Autodesk Inventor part; units mm, degrees
ref_plane "YZ Plane" through (0, 0, 0) normal (1, 0, 0) x (0, 1, 0)
ref_plane "XZ Plane" through (0, 0, 0) normal (0, 1, 0) x (-1, 0, 0)
ref_plane "XY Plane" through (0, 0, 0) normal (0, 0, 1) x (1, 0, 0)
sketch "スケッチ1" plane through (0, 0, 0) normal (0, 1, 0) x (-1, 0, 0)
  circle A0 centre (0, 0) radius 4
  dimension "d0" = 8
extrude "押し出し1" add sketch "スケッチ1" along normal blind 5
fillet "フィレット1" radius 0.2 1 edges at (4, 5, 0)
fillet "フィレット2" radius 0.2 1 edges at (4, 0, 0)
sketch "スケッチ2" plane through (0, 5, 0) normal (0, 1, 0) x (1, 0, 0)
  circle A0 centre (0, 0) radius 2
  dimension "d5" = 4
extrude "押し出し2" cut sketch "スケッチ2" against normal blind 5
sketch "スケッチ3" plane through (0, 0, 0) normal (0, 0, 1) x (1, 0, 0)
  line L0 (3.8, 0) -> (-3.8, 0)
  point P0 (0, 0)
  point P1 (0, 2.5)
  dimension "d8" = 2.5
hole "穴1" at (0, 2.5, 0) direction (0, 0, -1) diameter 2.459 depth 5 tip angle 118
properties part number "シャフトカラー" material "ステンレス鋼"
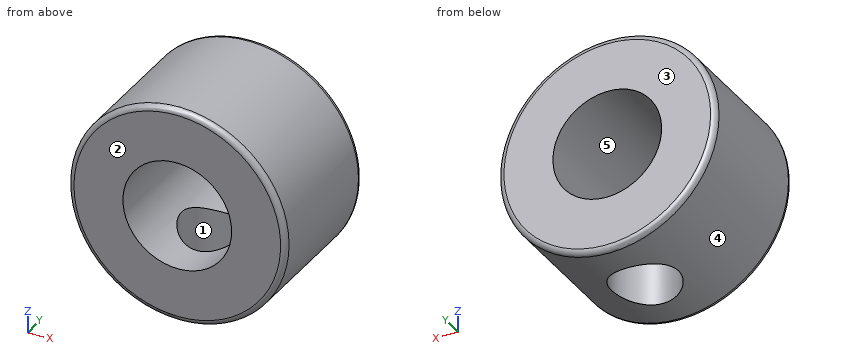
CAD build for the part. Positions are in the model's coordinates, mm. Face numbers are marked on the shaded views. A direction names the side the tool comes from. Round coordinates to 2 decimals unless told otherwise and drop trailing zeros. Order: outer loops, then holes, each group sorted by start corner. A loop starts at its lowest first (then second) coordinate and runs counter-clockwise, first axis right, second up. Notation, with made-up numbers: (34, 57.25) -> (69, 57.25) arc R8 cw to (69, 67.25) -> close; hole circle Ø8 at (38, 4.25). An arc over 180 degrees is marked (long way). One line per question, with ' | ' between items.
Q1. Two-plate mould, pull along X, no slides. Class the marked faces 3, 4 and 5: released by +X, released by -X, zero draft, split by the parting line, or undercut.
Completed:
face 3: zero draft | face 4: split by the parting line | face 5: undercut
Q2. Drop flat-ended pins along their axis: pin 1 (4.5 mm diameter, centred on x = 0, z = 0, fed in from -Y); pin 2 (2 mm diameter, centred on x = -2, y = 2.5, fed in from -Z); pin 3 (1 mm diameter, centred on y = 3.5, z = -3, fed in from +X); pin 4 (1 mm diameter, centred on y = 2, z = -3, fed in from -X). Give the stop position or say it passes through.
Completed:
pin 1: stops at y = 0 | pin 2: stops at z = -3.84 | pin 3: stops at x = 3.12 | pin 4: stops at x = -3.12
Q3. Slice it at C-C (y = 3.9). Write the cut outline in (x, z).
Completed:
outline: circle Ø8 at (0, 0); hole circle Ø4 at (0, 0)
Q4. Slice it at A-A (x = 0). Write the cut outline in (y, z), then the cut area to 3 significant figures.
Completed:
outline: (0, -3.8) arc R0.2 ccw to (0.2, -4) -> (1.27, -4) -> (1.27, -2) -> (0, -2) -> close; (0, 2) -> (5, 2) -> (5, 3.8) arc R0.2 ccw to (4.8, 4) -> (0.2, 4) arc R0.2 ccw to (0, 3.8) -> close; (3.73, -4) -> (4.8, -4) arc R0.2 ccw to (5, -3.8) -> (5, -2) -> (3.73, -2) -> close | area: 15.0 mm^2
Q5. Probe probe 1 along Y at (x, z) = (0, -2.65); probe 2 along Z at (x, y) = (0, 1.6); probe 3 along Z at (x, y) = (1.25, 3.75). List the from-to ranges inside material, lowest first.
Completed:
probe 1: y = 0 to 1.27, 3.73 to 5 | probe 2: z = 2 to 4 | probe 3: z = -3.8 to -1.56, 1.56 to 3.8
Q6. Which spindle directions (+Z, -Z, +X, -X, +Y, -Y) get a long thin tool onto all of the face, cutting with end or side? Do the marked faces 1 and 2. Say none if no direction does.
Completed:
face 1: -Z | face 2: +Z, -Z, +X, -X, -Y
Q7. Slice it at B-B (z = 0). Write the cut outline in (x, y).
Completed:
outline: (-4, 0.2) arc R0.2 ccw to (-3.8, 0) -> (-2, 0) -> (-2, 5) -> (-3.8, 5) arc R0.2 ccw to (-4, 4.8) -> close; (2, 0) -> (3.8, 0) arc R0.2 ccw to (4, 0.2) -> (4, 4.8) arc R0.2 ccw to (3.8, 5) -> (2, 5) -> close
Q8. Slice it at D-D (y = 1.75). Write the cut outline in (x, z).
Completed:
outline: (-0.97, -3.88) -> (-0.97, -1.75) arc R2 cw (long way) to (0.97, -1.75) -> (0.97, -3.88) arc R4 ccw (long way) to start
